Can you work these out from the model? Positions are in its coordinate system, mm. A direction names the side the tool comes from. Coordinates: 2 decimals unless noted, no trailing zeros. Order: outer loops, then holes, each group sorted by start corner. A loop starts at its lowest first (then second) coordinate and runs counter-clockwise, first axis right, second up. Notation, with made-up numbers: (-11, -32.5) -> (8, -32.5) arc R31 ccw to (8, 5.5) -> close; hole circle Ø4 at (-34.75, 35.25). An arc over 180 degrees is marked (long way). Answer as CSV lines item,"result".
from build123d import *

# Parameters (mm, degrees)
F0_R          = 19.05
F1_DEPTH      = 50.8
F2_W          = 101.6
F2_H          = 254
F3_DEPTH      = 101.6
F5_DEPTH      = 150.00483
F7_DEPTH      = 133.96625
F8_SIZE       = 25.39999
F9_T1_DEPTH   = 70.526940908
F9_T3_DEPTH   = 70.526940908
F10_T1_DEPTH  = 69.1227672529
F10_T3_DEPTH  = 191.4591513789
F10_T5_DEPTH  = 70.526940908
F10_T7_DEPTH  = 68.974059705
F10_T9_DEPTH  = 70.526940908
F11_T4_DEPTH  = 191.4591513789
F11_T9_DEPTH  = 191.4591513789
F11_T14_DEPTH = 191.4591513789
F11_T19_DEPTH = 191.4591513789
F13_R         = 12.7
F14_DEPTH     = 159.81291
F15_W         = 344.3993236951
F15_H         = 25.4
F16_DEPTH     = 6.35
F17_W         = 344.3993236951
F17_H         = 25.4
F18_DEPTH     = 6.35
F19_T1_DEPTH  = 25.4
F21_DEPTH     = 157.5482


# Not quite as in the source:
# - a fillet or chamfer that OpenCascade refuses, or shapes differently, is made with other operations: its cross-section is extruded or revolved along the edge and cut away or added
# - a fillet or chamfer is up to 0.001 mm smaller than in the source, because OpenCascade refuses the exact size
# - a feature of the source that left no trace in its solid (it failed there, or was rolled back) is left out


with BuildPart() as f1:
    # F0 (on Front) → F1 (new body)
    with BuildSketch(Plane.XZ):
        with BuildLine():
            ThreePointArc((-214.4006763049, -25.4), (-127.8432927657, -37.9486366929), (-48.4130559398, -74.5612903226))
            ThreePointArc((-48.4130559398, -74.5612903226), (88.9, 0), (-48.4130559398, 74.5612903226))
            ThreePointArc((-48.4130559398, 74.5612903226), (-127.8432927657, 37.9486366929), (-214.4006763049, 25.4))
            Line((-214.4006763049, 25.4), (-558.8, 25.4))
            Line((-558.8, 25.4), (-558.8, -25.4))
            Line((-558.8, -25.4), (-214.4006763049, -25.4))
        make_face()
        Circle(F0_R, mode=Mode.SUBTRACT)
    extrude(amount=F1_DEPTH)

    # F2 (on face) → F3 (join)
    with BuildSketch(Plane(origin=(-558.8, 0, 0), x_dir=(0, -1, 0), z_dir=(-1, 0, 0))):
        with Locations((25.4, -25.4)):
            Rectangle(F2_W, F2_H)
    extrude(amount=F3_DEPTH)

    # F4 (on face) → F5 (cut)
    with BuildSketch(Plane(origin=(0, 25.4, 0), x_dir=(-1, 0, 0), z_dir=(0, 1, 0))):
        Polygon((534.5858503342, 124.7548833489), (558.8, 44.7322204709), (609.6, 101.6), (660.4, 44.7322204709), (660.4, 124.7548833489), align=None)
    extrude(amount=-F5_DEPTH, mode=Mode.SUBTRACT)

    # F6 (on face) → F7 (cut)
    with BuildSketch(Plane(origin=(-660.4, 0, 0), x_dir=(0, -1, 0), z_dir=(-1, 0, 0))):
        Polygon((-36.009144038, 107.4853688478), (-25.4, 44.7322204709), (25.4, 100.9804829955), (76.2, 44.7322204709), (85.7249945402, 107.4853688478), align=None)
    extrude(amount=-F7_DEPTH, mode=Mode.SUBTRACT)

    # F8 (size 25.4 in the source; OpenCascade refuses exactly that, so slightly less here)
    f8_edges = [f1.edges().sort_by_distance(p)[0] for p in [
        (-660.4, -76.2, -53.83389),
        (-558.8, -76.2, -53.83389),
        (-558.8, 25.4, -53.83389),
        (-660.4, 25.4, -53.83389),
        (-609.6, 25.4, -152.4),
        (-609.6, -76.2, -152.4),
        (-558.8, -25.4, -152.4),
        (-660.4, -25.4, -152.4),
    ]]
    chamfer(f8_edges, length=F8_SIZE)

    # F9: fillet of radius 9.525 on 4 edges, made by hand

    # F9_s2 → F9_t1 (cut)
    with BuildSketch(Plane.YZ.offset(-644.863470454)):
        with BuildLine():
            ThreePointArc((2.7898179092, -149.6101920908), (-0.3003144883, -151.6749525472), (-3.9453741816, -152.4))
            Line((-3.9453741816, -152.4), (1e-05, -152.4))
            Line((1e-05, -152.4), (2.7898179092, -149.6101920908))
        make_face()
        with BuildLine():
            ThreePointArc((-53.5898179092, -149.6101920908), (-50.4996855117, -151.6749525472), (-46.8546258184, -152.4))
            Line((-46.8546258184, -152.4), (-50.80001, -152.4))
            Line((-50.80001, -152.4), (-53.5898179092, -149.6101920908))
        make_face()
    extrude(amount=F9_T1_DEPTH, mode=Mode.SUBTRACT)

    # F9_s4 → F9_t3 (cut)
    with BuildSketch(Plane.XZ.offset(-9.863470454)):
        with BuildLine():
            ThreePointArc((-581.4101820908, -149.6101920908), (-584.5003144883, -151.6749525472), (-588.1453741816, -152.4))
            Line((-588.1453741816, -152.4), (-584.19999, -152.4))
            Line((-584.19999, -152.4), (-581.4101820908, -149.6101920908))
        make_face()
        with BuildLine():
            ThreePointArc((-631.0546258184, -152.4), (-634.6996855117, -151.6749525472), (-637.7898179092, -149.6101920908))
            Line((-637.7898179092, -149.6101920908), (-635.00001, -152.4))
            Line((-635.00001, -152.4), (-631.0546258184, -152.4))
        make_face()
    extrude(amount=F9_T3_DEPTH, mode=Mode.SUBTRACT)

    # F10: fillet of radius 9.525 on 12 edges, made by hand

    # F10_s2 → F10_t1 (cut)
    with BuildSketch(Plane.YZ.offset(-644.1613836265)):
        with BuildLine():
            ThreePointArc((-73.7438328649, 47.4518097193), (-75.5647766574, 44.4878312477), (-76.2, 41.0676710203))
            Line((-76.2, 41.0676710203), (-76.2, 44.7322204709))
            Line((-76.2, 44.7322204709), (-73.7438328649, 47.4518097193))
        make_face()
        with BuildLine():
            ThreePointArc((22.9438328649, 47.4518097193), (24.7647766574, 44.4878312477), (25.4, 41.0676710203))
            Line((25.4, 41.0676710203), (25.4, 44.7322204709))
            Line((25.4, 44.7322204709), (22.9438328649, 47.4518097193))
        make_face()
    extrude(amount=F10_T1_DEPTH, mode=Mode.SUBTRACT)

    # F10_s4 → F10_t3 (cut)
    with BuildSketch(Plane.XY.offset(-136.863470454)):
        with BuildLine():
            ThreePointArc((-637.7898179092, -73.4101920908), (-634.6996855117, -75.4749525472), (-631.0546258184, -76.2))
            Line((-631.0546258184, -76.2), (-635.00001, -76.2))
            Line((-635.00001, -76.2), (-637.7898179092, -73.4101920908))
        make_face()
        with BuildLine():
            ThreePointArc((-581.4101820908, -73.4101920908), (-584.5003144883, -75.4749525472), (-588.1453741816, -76.2))
            Line((-588.1453741816, -76.2), (-584.19999, -76.2))
            Line((-584.19999, -76.2), (-581.4101820908, -73.4101920908))
        make_face()
        with BuildLine():
            ThreePointArc((-637.7898179092, 22.6101920908), (-634.6996855117, 24.6749525472), (-631.0546258184, 25.4))
            Line((-631.0546258184, 25.4), (-635.00001, 25.4))
            Line((-635.00001, 25.4), (-637.7898179092, 22.6101920908))
        make_face()
        with BuildLine():
            ThreePointArc((-581.4101820908, 22.6101920908), (-584.5003144883, 24.6749525472), (-588.1453741816, 25.4))
            Line((-588.1453741816, 25.4), (-584.19999, 25.4))
            Line((-584.19999, 25.4), (-581.4101820908, 22.6101920908))
        make_face()
        with BuildLine():
            ThreePointArc((-657.6101920908, 2.7898179092), (-659.6749525472, -0.3003144883), (-660.4, -3.9453741816))
            Line((-660.4, -3.9453741816), (-660.4, 1e-05))
            Line((-660.4, 1e-05), (-657.6101920908, 2.7898179092))
        make_face()
        with BuildLine():
            ThreePointArc((-657.6101920908, -53.5898179092), (-659.6749525472, -50.4996855117), (-660.4, -46.8546258184))
            Line((-660.4, -46.8546258184), (-660.4, -50.80001))
            Line((-660.4, -50.80001), (-657.6101920908, -53.5898179092))
        make_face()
    extrude(amount=F10_T3_DEPTH, mode=Mode.SUBTRACT)

    # F10_s6 → F10_t5 (cut)
    with BuildSketch(Plane.YZ.offset(-644.863470454)):
        with BuildLine():
            ThreePointArc((-76.2, -123.0546258184), (-75.4749525472, -126.6996855117), (-73.4101920908, -129.7898179092))
            Line((-73.4101920908, -129.7898179092), (-76.2, -127.00001))
            Line((-76.2, -127.00001), (-76.2, -123.0546258184))
        make_face()
        with BuildLine():
            ThreePointArc((25.4, -123.0546258184), (24.6749525472, -126.6996855117), (22.6101920908, -129.7898179092))
            Line((22.6101920908, -129.7898179092), (25.4, -127.00001))
            Line((25.4, -127.00001), (25.4, -123.0546258184))
        make_face()
    extrude(amount=F10_T5_DEPTH, mode=Mode.SUBTRACT)

    # F10_s8 → F10_t7 (cut)
    with BuildSketch(Plane.XZ.offset(-9.0870298525)):
        with BuildLine():
            ThreePointArc((-657.9784923634, 47.4429638254), (-659.7740558421, 44.4933557154), (-660.4, 41.0974125299))
            Line((-660.4, 41.0974125299), (-660.4, 44.7322204709))
            Line((-660.4, 44.7322204709), (-657.9784923634, 47.4429638254))
        make_face()
    extrude(amount=F10_T7_DEPTH, mode=Mode.SUBTRACT)

    # F10_s10 → F10_t9 (cut)
    with BuildSketch(Plane.XZ.offset(-9.863470454)):
        with BuildLine():
            ThreePointArc((-660.4, -123.0546258184), (-659.6749525472, -126.6996855117), (-657.6101920908, -129.7898179092))
            Line((-657.6101920908, -129.7898179092), (-660.4, -127.00001))
            Line((-660.4, -127.00001), (-660.4, -123.0546258184))
        make_face()
    extrude(amount=F10_T9_DEPTH, mode=Mode.SUBTRACT)

    # F11: fillet of radius 9.525 on 2 edges, made by hand


with BuildPart() as f11_tool2:
    # F11_s3 → F11_t4 (new body)
    with BuildSketch(Plane.XY.offset(-136.863470454)):
        with BuildLine():
            ThreePointArc((-558.8, -46.8546258184), (-559.5250474528, -50.4996855117), (-561.5898079092, -53.5898179092))
            Line((-561.5898079092, -53.5898179092), (-558.8, -50.80001))
            Line((-558.8, -50.80001), (-558.8, -46.8546258184))
        make_face()
    extrude(amount=F11_T4_DEPTH)

    split(bisect_by=Plane.XY.offset(-25.4), keep=Keep.BOTTOM)


with BuildPart() as f1_1:
    add(f1.part)

    # F11_t1: cut F11_tool2
    add(f11_tool2.part, mode=Mode.SUBTRACT)


with BuildPart() as f11_tool7:
    # F11_s8 → F11_t9 (new body)
    with BuildSketch(Plane.XY.offset(-136.863470454)):
        with BuildLine():
            ThreePointArc((-558.8, -46.8546258184), (-559.5250474528, -50.4996855117), (-561.5898079092, -53.5898179092))
            Line((-561.5898079092, -53.5898179092), (-558.8, -50.80001))
            Line((-558.8, -50.80001), (-558.8, -46.8546258184))
        make_face()
    extrude(amount=F11_T9_DEPTH)

    split(bisect_by=Plane.XY.offset(25.4), keep=Keep.TOP)


with BuildPart() as f1_2:
    add(f1_1.part)

    # F11_t6: cut F11_tool7
    add(f11_tool7.part, mode=Mode.SUBTRACT)


with BuildPart() as f11_tool12:
    # F11_s13 → F11_t14 (new body)
    with BuildSketch(Plane.XY.offset(54.5956809249)):
        with BuildLine():
            ThreePointArc((-561.5898079092, 2.7898179092), (-559.5250474528, -0.3003144883), (-558.8, -3.9453741816))
            Line((-558.8, -3.9453741816), (-558.8, 1e-05))
            Line((-558.8, 1e-05), (-561.5898079092, 2.7898179092))
        make_face()
    extrude(amount=-F11_T14_DEPTH)

    split(bisect_by=Plane.XY.offset(25.4), keep=Keep.TOP)


with BuildPart() as f1_3:
    add(f1_2.part)

    # F11_t11: cut F11_tool12
    add(f11_tool12.part, mode=Mode.SUBTRACT)


with BuildPart() as f11_tool17:
    # F11_s18 → F11_t19 (new body)
    with BuildSketch(Plane.XY.offset(54.5956809249)):
        with BuildLine():
            ThreePointArc((-561.5898079092, 2.7898179092), (-559.5250474528, -0.3003144883), (-558.8, -3.9453741816))
            Line((-558.8, -3.9453741816), (-558.8, 1e-05))
            Line((-558.8, 1e-05), (-561.5898079092, 2.7898179092))
        make_face()
    extrude(amount=-F11_T19_DEPTH)

    split(bisect_by=Plane.XY.offset(-25.4), keep=Keep.BOTTOM)


with BuildPart() as f1_4:
    add(f1_3.part)

    # F11_t16: cut F11_tool17
    add(f11_tool17.part, mode=Mode.SUBTRACT)

    # F13 (on face) → F14 (cut)
    with BuildSketch(Plane(origin=(0, 0, -152.4), x_dir=(1, 0, 0), z_dir=(0, 0, -1))):
        with Locations((-609.6, 25.4)):
            Circle(F13_R)
    extrude(amount=-F14_DEPTH, mode=Mode.SUBTRACT)

    # F15 (on face) → F16 (cut)
    with BuildSketch(Plane.XY.offset(25.4)):
        with Locations((-386.6003381525, -25.4)):
            Rectangle(F15_W, F15_H)
    extrude(amount=-F16_DEPTH, mode=Mode.SUBTRACT)

    # F17 (on face) → F18 (cut)
    with BuildSketch(Plane(origin=(0, 0, -25.4), x_dir=(1, 0, 0), z_dir=(0, 0, -1))):
        with Locations((-386.6003381525, 25.4)):
            Rectangle(F17_W, F17_H)
    extrude(amount=-F18_DEPTH, mode=Mode.SUBTRACT)

    # F19: chamfer of 6.35 on 6 edges, made by hand

    # F19_s2 → F19_t1 (cut)
    with BuildSketch(Plane.XZ.offset(12.7)):
        with BuildLine():
            Line((-208.1802681416, -25.4634801631), (-214.4006763049, -19.1148026665))
            Line((-214.4006763049, -19.1148026665), (-214.4006763049, -25.4))
            ThreePointArc((-214.4006763049, -25.4), (-211.2004813817, -25.4168004098), (-208.1802681416, -25.4634801631))
        make_face()
        with BuildLine():
            Line((-208.1802681416, 25.4634801631), (-214.4006763049, 19.1148026665))
            Line((-214.4006763049, 19.1148026665), (-214.4006763049, 25.4))
            ThreePointArc((-214.4006763049, 25.4), (-211.2004813817, 25.4168004098), (-208.1802681416, 25.4634801631))
        make_face()
    extrude(amount=F19_T1_DEPTH, mode=Mode.SUBTRACT)

    # F20 (on face) → F21 (join)
    with BuildSketch(Plane(origin=(0, 0, 7.41291), x_dir=(1, 0, 0), z_dir=(0, 0, -1))):
        Polygon((-613.0348443985, 25.984024629), (-626.3800263405, 31.7753516138), (-628.3944249153, 25.984024629), align=None)
        Polygon((-591.8838977814, 23.9696521312), (-606.2363386154, 24.2214500904), (-591.8838977814, 17.4229387194), align=None)
    extrude(amount=F21_DEPTH)


solid = f1_4.part
Q1. Which directions (+Z, -Z, +X, -X, +Y, -Y) give clear straight access to the entire face, cutting with the end or side of a thin tool? Please do faces 5 (the flat face through (-168, -50.8, 1)), 6 (the flat face through (-610.13, -54.61, 68.64)), 7 (the flat face through (-647.6, -25, -139.8)), 8 (the cylindrical face through (-618.96, -33.983, -73.612)), 9 (the flat face through (-600, -35, -152.4)).
Solution:
face 5,"+Z, -Z, +X, -Y"
face 6,"+Z, -X, -Y"
face 7,"-Z, -X, +Y, -Y"
face 8,"-Z"
face 9,"-Z, +X, -X, +Y, -Y"
Q2. Imagine slicing it at A-A (z = 0). Give the number of separate pieces and of enclosed holes in the cut face, and give its area (3 significant figures).
Solution:
separate pieces,"2"
enclosed holes,"1"
area,"39,500 mm2"
Q3. For P1, Ø1, axis at x = -122.5, y = -50, coming from the -Z side; P2, Ø21.5, axis at y = -30.5, z = -58.5, coming from the +X side; P3, Ø2, axis at y = -15, z = 7.5, coming from the +X side, each with a flat end and sliding along its axis, tell me the tip position at first contact or that it passes through.
Solution:
P1,"z = -39.74"
P2,"x = 74.99"
P3,"x = 88.66"
Q4. If I drill on line 1 (Y direction, x = -609.6, z = -83); line 2 (X direction, y = -25.4, z = -69.5); line 3 (Z direction, x = 0, y = -25), over which ranges is the centre line in solid material (lowest first)?
Solution:
line 1,"-76.2 to -38.1, -12.7 to 25.4"
line 2,"-660.4 to -622.3, -596.9 to -558.8, -56.48 to 55.43"
line 3,"-88.9 to -19.05, 19.05 to 88.9"
Q5. Imagine slicing it at C-C (z = 81). List the corners of the cut face in (x, y) for me, and give its area (3 significant figures).
Solution:
outline,"(-628, -43.45) -> (-591.2, -43.45) -> (-591.2, -7.35) -> (-628, -7.35) -> close; (-36.64, -50.8) -> (36.64, -50.8) -> (36.64, 0) -> (-36.64, 0) -> close"
area,"5,050 mm2"
Q6. Imagine slicing it at D-D (x = -260.5). List the corners of the cut face in (y, z) for me.
Solution:
outline,"(-50.8, -25.4) -> (-38.1, -25.4) -> (-38.1, -19.05) -> (-12.7, -19.05) -> (-12.7, -25.4) -> (0, -25.4) -> (0, 25.4) -> (-12.7, 25.4) -> (-12.7, 19.05) -> (-38.1, 19.05) -> (-38.1, 25.4) -> (-50.8, 25.4) -> close"
Q7. Imagine slicing it at B-B (x = 0). List the corners of the cut face in (y, z) for me, and give its area (3 significant figures).
Solution:
outline,"(-50.8, -88.9) -> (0, -88.9) -> (0, -19.05) -> (-50.8, -19.05) -> close; (-50.8, 19.05) -> (0, 19.05) -> (0, 88.9) -> (-50.8, 88.9) -> close"
area,"7,100 mm2"
Q8. We'd pull the mould along Y, two halves only. Please class faces 1 (the flat face through (-390, -7, 25.4)), 2 (the flat face through (-389, -26, -19.05)), 3 (the flat face through (-642.9, -59, -136.3)), 4 (the flat face through (-558.8, -25, 32)): pulls with the +Y half, pulls with the -Y half, needs draft (parallel to the pull), parting line crosses it, or undercut.
Solution:
face 1,"needs draft"
face 2,"undercut"
face 3,"pulls with the -Y half"
face 4,"undercut"
